Autodesk Inventor part; units mm, degrees
ref_plane "YZ Plane" through (0, 0, 0) normal (1, 0, 0) x (0, 1, 0)
ref_plane "XZ Plane" through (0, 0, 0) normal (0, 1, 0) x (-1, 0, 0)
ref_plane "XY Plane" through (0, 0, 0) normal (0, 0, 1) x (1, 0, 0)
sketch "スケッチ1" plane through (0, 0, 0) normal (0, 0, 1) x (1, 0, 0)
  line L0 (0, 0) -> (10, 0)
  line L1 (10, 0) -> (10, 27)
  line L2 (10, 27) -> (0, 27)
  line L3 (0, 27) -> (0, 0)
  dimension "d0" = 27
  dimension "d1" = 10
extrude "押し出し1" add sketch "スケッチ1" along normal blind 10.273
sketch "スケッチ2" plane through (0, 0, 10.273) normal (0, 0, 1) x (1, 0, 0)
  line L0 (0, 27) -> (0, 0)
  line L1 (0, 13.5) -> (10, 13.5)
  line L2 (10, 0) -> (10, 27)
  line L3 (10, 27) -> (0, 27)
  line L4 (5, 27) -> (5, 0)
  line L5 (0, 0) -> (10, 0)
  line L6 (0, 27) -> (10, 27)
  point P0 (5, 23.5)
  point P1 (5, 3.5)
  dimension "d4" = 10
hole "穴1" at (5, 23.5, 10.273) at (5, 3.5, 10.273) direction (0, 0, -1) diameter 3.1 end through all
fillet "フィレット1" radius 5 4 edges at (0, 27, 5.1365) (10, 27, 5.1365) (10, 0, 5.1365) (0, 0, 5.1365)
properties part number "link1part2" material "アルミニウム 6061"
Verification items for the finished model (mm, model axes). Give positions to 0.01 mm unless a question says otherwise; leave off trailing zeros. Order: outer loops, then holes, each group sorted by start corner. A loop starts at its lowest first (then second) coordinate and runs counter-clockwise, first axis right, second up. Notation, with made-up numbers: M -31,-28 L 14,-28 A31 cw 14,11 Z; hole C -30,57.25 d8. An arc over 180 degrees is marked long. Return JSON: item names as keys, results as strings. Group by question number.
1) Scan lines: line 1 (Y direction, x = 5, z = 5.75); line 2 (X direction, y = 23.5, z = 4); line 3 (X direction, y = 3, z = 0.5). Record each from-to range of solid material in increasing order.
2) Go/stop test with flat-tipped pins: pin 1 Ø4 at (x, y) = (2.5, 13) entering from -Z; pin 2 Ø1.9 at (x, y) = (5, 3.5) entering from +Z; pin 3 Ø1 at (x, z) = (7, 6) entering from -Y. Record where each tip stops, or that it passes through.
3) Section check C-C on x = 6. Record the cut outline in (y, z).
4) Section check D-D on x = 1. Record the cut outline in (y, z), and give its area (3 significant figures).
5) Mould release check, pull along X, two halves, no side actions. Record for faces 1 (the face through (9, 25, 5)), 2 (the face through (4.93, 5.05, 5.06)), 3 (the face through (5, 14, 10.273)): pulls with the +X half, pulls with the -X half, needs draft (parallel to the pull), parting line crosses it, or undercut.
6) Section check B-B on y = 3. Record the cut outline in (x, z).
7) Section check A-A on z = 3.5. Give the number of separate pieces and of enclosed holes in the cut face, and give its area (3 significant figures).
Answer block:
{
 "1": {"line 1": "y = 0 to 1.95, 5.05 to 21.95, 25.05 to 27", "line 2": "x = 0.23 to 3.45, 6.55 to 9.77", "line 3": "x = 0.42 to 3.53, 6.47 to 9.58"},
 "2": {"pin 1": "stops at z = 0", "pin 2": "passes through", "pin 3": "stops at y = 0.23"},
 "3": {"outline": "M 0.1,0 L 2.32,0 L 2.32,10.27 L 0.1,10.27 Z; M 4.68,0 L 22.32,0 L 22.32,10.27 L 4.68,10.27 Z; M 24.68,0 L 26.9,0 L 26.9,10.27 L 24.68,10.27 Z"},
 "4": {"outline": "M 2,0 L 25,0 L 25,10.27 L 2,10.27 Z", "area": "236 mm^2"},
 "5": {"face 1": "pulls with the +X half", "face 2": "undercut", "face 3": "needs draft"},
 "6": {"outline": "M 0.42,0 L 3.53,0 L 3.53,10.27 L 0.42,10.27 Z; M 6.47,0 L 9.58,0 L 9.58,10.27 L 6.47,10.27 Z"},
 "7": {"separate pieces": "1", "enclosed holes": "2", "area": "233 mm^2"}
}
